```python
from build123d import *

# Parameters (mm, degrees)
F0_R     = 2.9845
F1_DEPTH = 7.62


with BuildPart() as f1:
    # F0 (on Top) → F1 (new body)
    with BuildSketch(Plane.XY):
        Polygon((-75.365749, 69.569385), (-113.465749, -51.580893), (13.534251, -51.580893), (140.534251, -51.580893), (102.434251, 69.569385), (13.534251, 69.569385), align=None)
        with Locations((-104.812158, -45.230893)):
            Circle(F0_R, mode=Mode.SUBTRACT)
        Polygon((-49.541476, -45.230893), (-100.24803, -45.230893), (-67.861694, -13.870002), (-52.485536, -38.758501), align=None, mode=Mode.SUBTRACT)
        Polygon((3.274268, -45.230893), (-40.41322, -45.230893), (-14.65364, -20.286936), align=None, mode=Mode.SUBTRACT)
        Polygon((-102.813653, -38.876052), (-85.852937, 15.055587), (-85.702804, 15.008373), (-71.278508, -8.339402), align=None, mode=Mode.SUBTRACT)
        Polygon((-63.202862, -9.358682), (-39.207877, 13.876552), (-18.399576, -15.075035), (-43.330528, -39.216602), (-44.222796, -40.080618), align=None, mode=Mode.SUBTRACT)
        Polygon((7.184251, 0.859504), (7.184251, -39.402304), (-9.878115, -15.662617), align=None, mode=Mode.SUBTRACT)
        with Locations((13.534251, -46.55671)):
            Circle(F0_R, mode=Mode.SUBTRACT)
        Polygon((23.794234, -45.230893), (41.722141, -20.286936), (67.481722, -45.230893), align=None, mode=Mode.SUBTRACT)
        with Locations((131.88066, -45.230893)):
            Circle(F0_R, mode=Mode.SUBTRACT)
        Polygon((127.316531, -45.230893), (76.609978, -45.230893), (79.554038, -38.758501), (94.930195, -13.870002), align=None, mode=Mode.SUBTRACT)
        Polygon((19.884251, -39.402304), (19.884251, 0.859504), (36.946616, -15.662617), align=None, mode=Mode.SUBTRACT)
        Polygon((45.468077, -15.075035), (66.276379, 13.876552), (90.271363, -9.358682), (71.291298, -40.080618), (70.39903, -39.216602), align=None, mode=Mode.SUBTRACT)
        Polygon((98.34701, -8.339402), (112.771306, 15.008373), (129.882154, -38.876052), align=None, mode=Mode.SUBTRACT)
        Polygon((-83.30042, 23.172075), (-71.91322, 59.381063), (-42.953813, 19.088452), (-66.619676, -3.828081), align=None, mode=Mode.SUBTRACT)
        Polygon((-34.432352, 18.50087), (7.184251, 58.799771), (7.184251, 9.698733), (-13.624051, -10.450717), align=None, mode=Mode.SUBTRACT)
        with Locations((-70.761945, 63.219385)):
            Circle(F0_R, mode=Mode.SUBTRACT)
        Polygon((-66.572778, 63.219385), (2.620123, 63.219385), (-38.178288, 23.71277), align=None, mode=Mode.SUBTRACT)
        Polygon((19.884251, 9.698733), (19.884251, 58.799771), (61.500854, 18.50087), (40.692552, -10.450717), align=None, mode=Mode.SUBTRACT)
        Polygon((70.022315, 19.088452), (98.981721, 59.381063), (110.368921, 23.172075), (93.688178, -3.828081), align=None, mode=Mode.SUBTRACT)
        Polygon((65.246789, 23.71277), (24.448379, 63.219385), (93.641279, 63.219385), align=None, mode=Mode.SUBTRACT)
        with Locations((13.534251, 64.711635)):
            Circle(F0_R, mode=Mode.SUBTRACT)
        with Locations((97.774625, 63.219385)):
            Circle(F0_R, mode=Mode.SUBTRACT)
    extrude(amount=F1_DEPTH)


solid = f1.part
```
The listing builds one solid part. Answer for the finished solid, in the listing's coordinates (mm). Coordinates: 2 decimals unless noted, no trailing zeros. Write each loop counter-clockwise with the first axis right and the second up, starting at its lowest first coordinate (ties: lowest second). Pieces come first, ordered by that corner, then holes. Notation, with made-up numbers: (35.25, -23.5) - (46.25, -23.5) arc R22 ccw to (46.25, -1.5) - close; hole circle Ø3 at (26, 7). An arc over 180 degrees is marked (long way). Return JSON: item names as keys, results as strings. Group by question number.
Q1. For a pull along Y with two mould halves and no side action, classify faces 1 (the flat face through (13, 0, 0)), 2 (the cylindrical face through (97.39, 66.18, 3.76)), 3 (the flat face through (-94.15, 9.84, 3.76)) as +Y half, -Y half, draft (parallel to the pull), parting line (faces both ways), or undercut.
Q2. The part is cut by section B-B on y = 55. Write down the section's boundary in (x, z).
Q3. The part is cut by section A-A on x = -6. Write down the section's boundary in (y, z), and give its area (3 significant figures).
Q4. The part is cut by section C-C on x = -59.5. Write down the section's boundary in (y, z).
Q5. The part is cut by section D-D on z = 1.25. State how many separate pieces and enclosed holes the cut face has, and give its area (3 significant figures).
Q6. Flat-ended cylindrical pins translate along their axes: pin 1 Ø4 at (y, z) = (43, 3.5) entering from +X; pin 2 Ø3 at (y, z) = (24.5, 6) entering from -X; pin 3 Ø1.5 at (y, z) = (-1, 2) entering from +X. Find the tip coordinate at first contact, or state that the pin passes through.
Q7. Find the intervals of material crossed by line 1 along Y through (x, z) = (52, 5); line 2 along Y through (x, z) = (54, 1.75); line 3 along Y through (x, z) = (-45.5, 5), in increasing order. Write a range as [from, to].
Evaluation:
{
 "1": {"face 1": "draft", "face 2": "undercut", "face 3": "+Y half"},
 "2": {"outline": "(-79.95, 0) - (-73.29, 0) - (-73.29, 7.62) - (-79.95, 7.62) - close; (-68.76, 0) - (-60.67, 0) - (-60.67, 7.62) - (-68.76, 7.62) - close; (-5.87, 0) - (3.26, 0) - (3.26, 7.62) - (-5.87, 7.62) - close; (7.18, 0) - (19.88, 0) - (19.88, 7.62) - (7.18, 7.62) - close; (23.81, 0) - (32.94, 0) - (32.94, 7.62) - (23.81, 7.62) - close; (87.73, 0) - (95.83, 0) - (95.83, 7.62) - (87.73, 7.62) - close; (100.36, 0) - (107.02, 0) - (107.02, 7.62) - (100.36, 7.62) - close"},
 "3": {"outline": "(-51.58, 0) - (-45.23, 0) - (-45.23, 7.62) - (-51.58, 7.62) - close; (-32.33, 0) - (-21.06, 0) - (-21.06, 7.62) - (-32.33, 7.62) - close; (-11.91, 0) - (-3.07, 0) - (-3.07, 7.62) - (-11.91, 7.62) - close; (46.03, 0) - (54.87, 0) - (54.87, 7.62) - (46.03, 7.62) - close; (63.22, 0) - (69.57, 0) - (69.57, 7.62) - (63.22, 7.62) - close", "area": "317 mm2"},
 "4": {"outline": "(-51.58, 0) - (-45.23, 0) - (-45.23, 7.62) - (-51.58, 7.62) - close; (-27.4, 0) - (-15.35, 0) - (-15.35, 7.62) - (-27.4, 7.62) - close; (-5.77, 0) - (3.07, 0) - (3.07, 7.62) - (-5.77, 7.62) - close; (42.11, 0) - (53.38, 0) - (53.38, 7.62) - (42.11, 7.62) - close; (63.22, 0) - (69.57, 0) - (69.57, 7.62) - (63.22, 7.62) - close"},
 "5": {"separate pieces": "1", "enclosed holes": "22", "area": "10,600 mm2"},
 "6": {"pin 1": "stops at x = 111.42", "pin 2": "stops at x = -90.01", "pin 3": "stops at x = 124.86"},
 "7": {"line 1": "y = [-51.58, -45.23], [-30.24, -21.4], [-5.99, 5.28], [27.7, 36.54], [63.22, 69.57]", "line 2": "y = [-51.58, -45.23], [-32.18, -23.34], [-3.2, 8.06], [25.76, 34.6], [63.22, 69.57]", "line 3": "y = [-51.58, -38.01], [7.78, 16.62], [22.63, 33.9], [63.22, 69.57]"}
}
